Geometry check sheet. Reference: the model listing, model coordinates, mm. Face numbers are marked on the shaded views. A direction names the side the tool comes from. Give positions to 0.01 mm unless a question says otherwise; leave off trailing zeros. Loops run counter-clockwise (first coordinate to the right, second up) from the corner with the lowest first, then second, coordinate; pieces in that order, holes last. Notation, with made-up numbers: (35, 72.5) -> (49, 72.5) arc R13 ccw to (49, 92.5) -> close; hole circle Ø11 at (4, 24). An arc over 180 degrees is marked (long way). Write each question's results on one line, items separated by ' | '. Start each with the question number.
1) Sectioned sample at A-A on y = 3. Record the cut outline in (x, z), then the cut area to 3 significant figures.
2) Sectioned sample at B-B on y = -12. Record the cut outline in (x, z), then the cut area to 3 significant figures.
3) Set-up check for the marked faces 1, 2 and 3: record each of +Z, -Z, +X, -X, +Y, -Y from which the full face is reachable in a straight line by a thin tool's end or side.
4) Scan lines: line 1 (X direction, y = -3.5, z = 0); line 2 (Y direction, x = 0.5, z = -5); line 3 (Z direction, x = -0.5, y = -18.5). Record each from-to range of solid material in increasing order. Write a range as from..to.
5) Depth check by flat-ended pin: pin 1 (6 mm diameter, centred on y = -18, z = 0, fed in from -X); pin 2 (6 mm diameter, centred on x = 1.5, y = -12, fed in from -Z); pin 3 (2 mm diameter, centred on x = -3, z = -3.5, fed in from -Y). Enter the tip coordinate at first touch or a pass-through.
```python
from build123d import *

# Parameters (mm, degrees)
BOSS_EXTRUDE1_DEPTH = 4
SKETCH2_OUTSIDE_W   = 29.082
SKETCH2_OUTSIDE_H   = 30.606
SKETCH2_OUTSIDE_R   = 5.014305997
CUT_EXTRUDE1_DEPTH  = 4
CUT_EXTRUDE1_DRAFT  = -60
SKETCH3_OUTSIDE_W   = 29.082
SKETCH3_OUTSIDE_H   = 30.606
SKETCH3_OUTSIDE_R   = 5.014305997
CUT_EXTRUDE2_DEPTH  = 4
CUT_EXTRUDE2_DRAFT  = -60
SKETCH4_R           = 3
BOSS_EXTRUDE3_DEPTH = 3
BOSS_EXTRUDE4_START = 30
SKETCH5_R           = 3
BOSS_EXTRUDE4_DEPTH = 30


with BuildPart() as part:
    # Sketch1 → Boss-Extrude1 (new body)
    with BuildSketch(Plane(origin=(0, 0, 0), x_dir=(1, 0, 0), z_dir=(0, 1, 0))):
        Polygon((5, 2.919649438), (-0.028490583, 5.789951738), (-5.028490583, 2.8703023), (-5, -2.919649438), (0.028490583, -5.789951738), (5.028490583, -2.8703023), align=None)
    extrude(amount=BOSS_EXTRUDE1_DEPTH)


with BuildPart() as cut_extrude1_tool:
    # Sketch2 outside → Cut-Extrude1 (with draft: the straight prism first)
    with BuildSketch(Plane(origin=(0, 4, 0), x_dir=(1, 0, 0), z_dir=(0, 1, 0))):
        Rectangle(SKETCH2_OUTSIDE_W, SKETCH2_OUTSIDE_H)
        Circle(SKETCH2_OUTSIDE_R, mode=Mode.SUBTRACT)
    extrude(amount=-CUT_EXTRUDE1_DEPTH)
    # Cut-Extrude1: the draft: its side faces are tilted about the plane it starts from
    cut_extrude1_sides = [cut_extrude1_tool.faces().sort_by_distance(p)[0] for p in [
        (0, 2, 15.303),
        (14.541, 2, 0),
        (0, 2, -15.303),
        (-14.541, 2, 0),
        (-5.014305997, 2, 0),
    ]]
    draft(cut_extrude1_sides, Plane(origin=(0, 4, 0), x_dir=(1, 0, 0), z_dir=(0, 1, 0)), CUT_EXTRUDE1_DRAFT)


with BuildPart() as part_1:
    add(part.part)

    # Cut-Extrude1: cut by cut_extrude1_tool
    add(cut_extrude1_tool.part, mode=Mode.SUBTRACT)


with BuildPart() as cut_extrude2_tool:
    # Sketch3 outside → Cut-Extrude2 (with draft: the straight prism first)
    with BuildSketch(Plane.XZ):
        Rectangle(SKETCH3_OUTSIDE_W, SKETCH3_OUTSIDE_H)
        Circle(SKETCH3_OUTSIDE_R, mode=Mode.SUBTRACT)
    extrude(amount=-CUT_EXTRUDE2_DEPTH)
    # Cut-Extrude2: the draft: its side faces are tilted about the plane it starts from
    cut_extrude2_sides = [cut_extrude2_tool.faces().sort_by_distance(p)[0] for p in [
        (0, 2, -15.303),
        (14.541, 2, 0),
        (0, 2, 15.303),
        (-14.541, 2, 0),
        (-5.014305997, 2, 0),
    ]]
    draft(cut_extrude2_sides, Plane.XZ, CUT_EXTRUDE2_DRAFT)


with BuildPart() as part_2:
    add(part_1.part)

    # Cut-Extrude2: cut by cut_extrude2_tool
    add(cut_extrude2_tool.part, mode=Mode.SUBTRACT)

    # Sketch4 → Boss-Extrude3 (add)
    with BuildSketch(Plane(origin=(0, 4, 0), x_dir=(1, 0, 0), z_dir=(0, 1, 0))):
        with Locations(Location((0, 0, 0), (0, 0, 270))):
            Circle(SKETCH4_R)
    extrude(amount=BOSS_EXTRUDE3_DEPTH)

    # Sketch5 → Boss-Extrude4 (add)
    with BuildSketch(Plane.XZ.offset(BOSS_EXTRUDE4_START)):
        with Locations(Location((0, 0, 0), (0, 0, 90))):
            Circle(SKETCH5_R)
    extrude(amount=-BOSS_EXTRUDE4_DEPTH)


solid = part_2.part
```
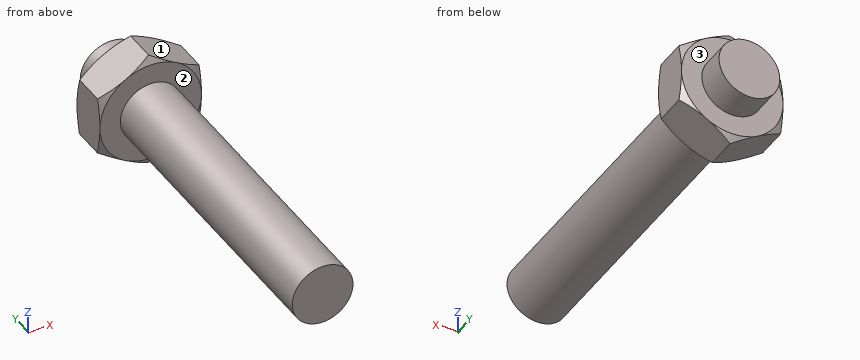
Result:
1) outline: (-5.03, -2.87) -> (-0.03, -5.79) -> (5, -2.92) -> (5.03, 2.87) -> (0.03, 5.79) -> (-5, 2.92) -> close | area: 87.1 mm^2
2) outline: circle Ø6 at (0, 0) | area: 28.3 mm^2
3) face 1: +Z, +X, +Y, -Y | face 2: -Y | face 3: +Y
4) line 1: -3..3 | line 2: 0.01..3.99 | line 3: -2.96..2.96
5) pin 1: x = -3 | pin 2: z = -3 | pin 3: y = 0
